Geometry: final body of the model. Coordinates: model frame, mm. A direction names the side the tool comes from. Give positions to 0.01 mm unless a question says otherwise; leave off trailing zeros. Write each loop counter-clockwise with the first axis right and the second up, starting at its lowest first coordinate (ties: lowest second). Pieces come first, ordered by that corner, then holes.
Q1. Section C-C (x = -10). Return the cut outline in (y, z).
Q2. Pin query (flat end, axial travel): pin 1 Ø2 at (x, y) = (-13, 3) entering from +Z; pin 2 Ø1 at (x, y) = (-7, 2) entering from -Z. Return the tip coordinate at first contact, or that it passes through.
Q3. Section B-B (y = 2.85). Return the cut outline in (x, z) (3 decimals), plus the area to 3 significant figures.
Q4. Section D-D (x = -6.5). Return the cut outline in (y, z), plus the area to 3 significant figures.
Q5. Reachability of faces 5 (the flat face through (-13.213, 2, 2)), 6 (the cylindrical face through (-6.66, 2.54, 32.31)) from +Z, -Z, +X, -X, +Y, -Y: full face, straight path, thin tool, end or side. Return the list, or none.
Q6. Section A-A (z = -3). Return the cut outline in (x, y), plus the area to 3 significant figures.
Q7. Mould query, pull axis Z, two halves, no side actions, for faces 1 (the cylindrical face through (-12.49, 2.54, 22.68)), 2 (the cylindrical face through (-13.02, 2.46, 28.75)), 3 (the cylindrical face through (-14.667, 2.535, -21.657)), 4 (the flat face through (-4.94, 2, 6)). Classes: +Z half, -Z half, draft (parallel to the pull), parting line (faces both ways), or undercut.
Q8. Line query: line 1 (X direction, y = 4.5, z = -1); line 2 (Z direction, x = -12, y = 2.45); line 3 (Z direction, x = -10, y = 4.7). Output: solid intervals per line, ascending.
Autodesk Inventor part; units mm, degrees
ref_plane "YZ Plane" through (0, 0, 0) normal (1, 0, 0) x (0, 1, 0)
ref_plane "XZ Plane" through (0, 0, 0) normal (0, 1, 0) x (-1, 0, 0)
ref_plane "XY Plane" through (0, 0, 0) normal (0, 0, 1) x (1, 0, 0)
sketch "Sketch1" plane through (0, 0, 0) normal (0, 1, 0) x (-1, 0, 0)
  line L0 (16.3851, 33.9368) -> (4.9404, 33.9368)
  line L1 (4.9404, 33.9368) -> (4.9404, -23.2869)
  line L2 (4.9404, -23.2869) -> (16.3851, -23.2869)
  line L3 (16.3851, -23.2869) -> (16.3851, 33.9368)
  line L4 (13.2127, 30.325) -> (8.1127, 30.325)
  line L5 (8.1127, 30.325) -> (8.1127, -19.675)
  line L6 (8.1127, -19.675) -> (13.2127, -19.675)
  line L7 (13.2127, -19.675) -> (13.2127, 30.325)
  circle A0 centre (10.6627, 27.775) radius 2.55
  line L8 (13.2127, 23.4447) -> (8.1127, 23.4447)
  point P0 (0, 0)
  dimension "d2" = 5.1
  dimension "d3" = 11.4447
  dimension "d4" = 57.2237
  dimension "d5" = 3.1724
  dimension "d6" = 50
  dimension "d7" = 3.6118
  dimension "d12" = 5.1
  dimension "d13" = 2.55
extrude "Extrusion2" add sketch "Sketch1" along normal blind 5 contours L3 L2 L1 L0 | L7 A0 L4 | A0 L5 L4 | L7 L8 L5 A0
fillet "Fillet3" radius 5.715 4 edges at (-16.3851, 2.5, 33.9368) (-4.9404, 2.5, 33.9368) (-16.3851, 2.5, -23.2869) (-4.9404, 2.5, -23.2869)
fillet "Fillet4" radius 2.54 4 edges at (-13.2127, 2.5, 23.4447) (-8.1127, 2.5, 23.4447) (-8.1127, 2.5, -19.675) (-13.2127, 2.5, -19.675)
equation "\"d5\" = -0.5 * d2 + 0.5 * d3"
equation "\"d7\" = -0.5 * d6 + 0.5 * d4"
equation "\"d12\" = d2"
equation "\"d13\" = 0.5 * d2"
properties part number "extention_plate"
Computed:
1. outline: (0, -23.25) - (5, -23.25) - (5, -19.59) - (0, -19.59) - close; (0, 23.36) - (5, 23.36) - (5, 25.31) - (0, 25.31) - close; (0, 30.24) - (5, 30.24) - (5, 33.9) - (0, 33.9) - close
2. pin 1: stops at z = 33.78
2. pin 2: stops at z = -22.34
3. outline: (-16.385, -17.572) arc R5.715 ccw to (-10.67, -23.287) - (-10.655, -23.287) arc R5.715 ccw to (-4.94, -17.572) - (-4.94, 28.222) arc R5.715 ccw to (-10.655, 33.937) - (-10.67, 33.937) arc R5.715 ccw to (-16.385, 28.222) - close; hole (-13.213, -17.135) arc R2.54 ccw to (-10.673, -19.675) - (-10.653, -19.675) arc R2.54 ccw to (-8.113, -17.135) - (-8.113, 20.905) arc R2.54 ccw to (-10.653, 23.445) - (-10.673, 23.445) arc R2.54 ccw to (-13.213, 20.905) - close; hole circle Ø5.1 at (-10.663, 27.775)
3. area: 392 mm2
4. outline: (0, -21.5) - (5, -21.5) - (5, 32.15) - (0, 32.15) - close
4. area: 268 mm2
5. face 5: +Y, -Y
5. face 6: +Z, +X, +Y, -Y
6. outline: (-16.39, 0) - (-13.21, 0) - (-13.21, 5) - (-16.39, 5) - close; (-8.11, 0) - (-4.94, 0) - (-4.94, 5) - (-8.11, 5) - close
6. area: 31.7 mm2
7. face 1: undercut
7. face 2: undercut
7. face 3: -Z half
7. face 4: draft
8. line 1: x = -16.39 to -13.21, -8.11 to -4.94
8. line 2: z = -23.13 to -19.3, 23.07 to 25.6, 29.95 to 33.78
8. line 3: z = -23.25 to -19.59, 23.36 to 25.31, 30.24 to 33.9
